Autodesk Inventor part; units mm, degrees
ref_plane "YZ Plane" through (0, 0, 0) normal (1, 0, 0) x (0, 1, 0)
ref_plane "XZ Plane" through (0, 0, 0) normal (0, 1, 0) x (-1, 0, 0)
ref_plane "XY Plane" through (0, 0, 0) normal (0, 0, 1) x (1, 0, 0)
sketch "Sketch1" plane through (0, 0, 0) normal (0, 1, 0) x (-1, 0, 0)
  line L0 (-11.43, -6.35) -> (11.43, -6.35)
  line L1 (11.43, -6.35) -> (11.43, 6.35)
  line L2 (11.43, 6.35) -> (-11.43, 6.35)
  line L3 (-11.43, 6.35) -> (-11.43, -6.35)
  line L4 (-11.43, -6.35) -> (11.43, 6.35) construction
  line L5 (11.43, -6.35) -> (-11.43, 6.35) construction
  point P0 (0, 0)
  point P1 (0, 0)
  dimension "d19" = 22.86
  dimension "d20" = 12.7
sketch "Sketch2" plane through (0, 0, 0) normal (0, 1, 0) x (-1, 0, 0)
  line L0 (9.525, 3.1634) -> (9.525, -3.1866) construction
  line L1 (9.525, -3.1866) -> (-9.525, -3.1866) construction
  line L2 (-9.525, -3.1866) -> (-9.525, 3.1634) construction
  line L3 (-9.525, 3.1634) -> (9.525, 3.1634) construction
  line L4 (9.525, 6.3268) -> (9.525, 3.1634) construction
  line L5 (-9.525, 3.1634) -> (-9.525, 6.5546) construction
  line L6 (11.43, -6.35) -> (11.43, 6.35)
  line L7 (-11.43, -6.35) -> (11.43, -6.35)
  line L8 (-11.43, 6.35) -> (-11.43, -6.35)
  line L9 (11.43, 6.35) -> (-11.43, 6.35)
  line L10 (9.525, -3.1866) -> (9.525, -6.35) construction
  point P0 (0, 0)
  dimension "d18" = 6.35
  dimension "d22" = 19.05
  dimension "d23" = 1.905
  dimension "d24" = 3.1634
extrude "Extrusion1" add sketch "Sketch1" along normal blind 5.08
hole "Hole1" at (-9.525, 0, 3.1634) at (-9.525, 0, -3.1866) at (9.525, 0, -3.1866) at (9.525, 0, 3.1634) direction (0, 1, 0) diameter 2.4384 depth 5.08
sketch "Sketch3" plane through (0, 0, 0) normal (0, -1, 0) x (1, 0, 0)
  line L0 (11.43, -6.35) -> (-11.43, -6.35)
  line L1 (7.62, 6.35) -> (-7.62, 6.35)
  line L2 (-7.62, 6.35) -> (-7.62, -6.35)
  line L3 (-7.62, -6.35) -> (7.62, -6.35)
  line L4 (7.62, -6.35) -> (7.62, 6.35)
  line L5 (7.62, 6.35) -> (-7.62, -6.35) construction
  line L6 (-7.62, 6.35) -> (7.62, -6.35) construction
  point P0 (0, 0)
  point P1 (7.62, -6.35)
  dimension "d34" = 15.24
extrude "Extrusion2" cut sketch "Sketch3" against normal blind 2.54
properties part number "Controller_Strap"
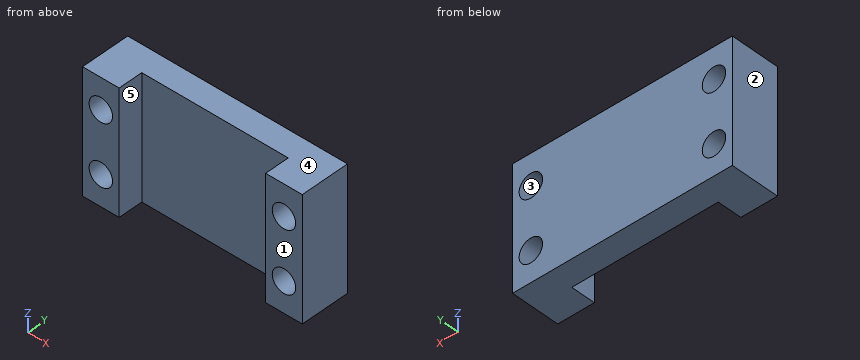
Model file for the job. Use its own axes, mm. Face numbers are marked on the shaded views. A direction names the side the tool comes from. Round coordinates to 2 decimals unless told otherwise and drop trailing zeros. Loops run counter-clockwise (first coordinate to the right, second up) from the corner with the lowest first, then second, coordinate; pieces in that order, holes last.
1. Drop flat-ended pins along their axis: P1, Ø2, axis at x = -9.52, z = -3.19, coming from the +Y side; P2, Ø1, axis at x = -5, y = 2.5, coming from the +Z side; P3, Ø4, axis at x = -5.5, z = 4.5, coming from the -Y side. Give the stop position or say it passes through.
Check values:
P1: passes through
P2: stops at z = 6.35
P3: stops at y = 2.54
2. Tool access for the marked faces 4 and 5: list every direction of +Z, -Z, +X, -X, +Y, -Y with a clear straight run to the whole face (end or side of a thin tool).
Check values:
face 4: +Z, +X, -X, +Y, -Y
face 5: +Z, -Z, -Y
3. Mould opens along X. For the marked faces 1, 2 and 3 say: +X half, -X half, draft (parallel to the pull), parting line (faces both ways), or undercut.
Check values:
face 1: draft
face 2: -X half
face 3: undercut
4. Band-saw the part on D-D, the plane x = -3.25. List the corners of the cut face in (y, z).
Check values:
outline: (2.54, -6.35) - (5.08, -6.35) - (5.08, 6.35) - (2.54, 6.35) - close
5. Band-saw the part on B-B, the plane y = 1.4. List the corners of the cut face in (x, z) (3 decimals).
Check values:
outline: (-11.43, -6.35) - (-7.62, -6.35) - (-7.62, 6.35) - (-11.43, 6.35) - close; (7.62, -6.35) - (11.43, -6.35) - (11.43, 6.35) - (7.62, 6.35) - close; hole circle Ø2.438 at (-9.525, -3.187); hole circle Ø2.438 at (-9.525, 3.163); hole circle Ø2.438 at (9.525, -3.187); hole circle Ø2.438 at (9.525, 3.163)
6. Band-saw the part on A-A, the plane z = -0.5. List the corners of the cut face in (x, y).
Check values:
outline: (-11.43, 0) - (-7.62, 0) - (-7.62, 2.54) - (7.62, 2.54) - (7.62, 0) - (11.43, 0) - (11.43, 5.08) - (-11.43, 5.08) - close
7. Wall check: probe 1 along X at (y, z) = (2.15, 3.25); probe 2 along X at (y, z) = (2.25, -5.5); probe 3 along X at (y, z) = (2.6, 4). Give the ranges that are in metal, low to high.
Check values:
probe 1: x = -11.43 to -10.74, -8.31 to -7.62, 7.62 to 8.31, 10.74 to 11.43
probe 2: x = -11.43 to -7.62, 7.62 to 11.43
probe 3: x = -11.43 to -10.41, -8.64 to 8.64, 10.41 to 11.43
8. Band-saw the part on C-C, the plane z = -2.25. List the corners of the cut face in (x, y).
Check values:
outline: (-11.43, 0) - (-10.31, 0) - (-10.31, 5.08) - (-11.43, 5.08) - close; (-8.74, 0) - (-7.62, 0) - (-7.62, 2.54) - (7.62, 2.54) - (7.62, 0) - (8.74, 0) - (8.74, 5.08) - (-8.74, 5.08) - close; (10.31, 0) - (11.43, 0) - (11.43, 5.08) - (10.31, 5.08) - close
